Build history of the part. All positions in model axes, mm. A direction names the side the tool comes from. Give positions to 0.01 mm unless a question says otherwise; leave off trailing zeros. Write each loop counter-clockwise with the first axis right and the second up, starting at its lowest first coordinate (ties: lowest second). Pieces come first, ordered by that corner, then holes. Notation, with made-up numbers: (-36.75, 35) - (-27.75, 35) arc R22 ccw to (-27.75, 64) - close; hole circle Ø6 at (32, 54.5). An arc over 180 degrees is marked (long way). Use one line per item in the form item = value. Start each with the question number.
from build123d import *

# Parameters (mm, degrees)
BOSS_EXTRUDE1_DEPTH          = 18
F_4_0_4_DIAMETER_HOLE1_D     = 4
F_4_0_4_DIAMETER_HOLE1_DEPTH = 30
F_4_0_4_DIAMETER_HOLE1_TIP   = 1.201721238
F_4_0_4_DIAMETER_HOLE2_D     = 4
F_4_0_4_DIAMETER_HOLE2_DEPTH = 30
F_4_0_4_DIAMETER_HOLE2_TIP   = 1.201721238


with BuildPart() as part:
    # Sketch1 → Boss-Extrude1 (new body)
    with BuildSketch(Plane.XY):
        Polygon((30, 35), (60, 5), (60, -35), (-60, -35), (-60, 35), align=None)
    extrude(amount=BOSS_EXTRUDE1_DEPTH)

    # Ø4.0 (4) Diameter Hole1
    with Locations(Plane.ZY.offset(60)):
        with Locations((9, 16), (9, -16)):
            Hole(F_4_0_4_DIAMETER_HOLE1_D / 2, depth=F_4_0_4_DIAMETER_HOLE1_DEPTH)
            with Locations((0, 0, -(F_4_0_4_DIAMETER_HOLE1_DEPTH + F_4_0_4_DIAMETER_HOLE1_TIP / 2))):  # 118° drill point
                Cone(0, F_4_0_4_DIAMETER_HOLE1_D / 2, F_4_0_4_DIAMETER_HOLE1_TIP, mode=Mode.SUBTRACT)

    # Ø4.0 (4) Diameter Hole2
    with Locations(Plane(origin=(0, -35, 0), x_dir=(-1, 0, 0), z_dir=(0, -1, 0))):
        with Locations((-35, -9), (20, -9)):
            Hole(F_4_0_4_DIAMETER_HOLE2_D / 2, depth=F_4_0_4_DIAMETER_HOLE2_DEPTH)
            with Locations((0, 0, -(F_4_0_4_DIAMETER_HOLE2_DEPTH + F_4_0_4_DIAMETER_HOLE2_TIP / 2))):  # 118° drill point
                Cone(0, F_4_0_4_DIAMETER_HOLE2_D / 2, F_4_0_4_DIAMETER_HOLE2_TIP, mode=Mode.SUBTRACT)


solid = part.part
(1) Which spindle directions (+Z, -Z, +X, -X, +Y, -Y) get a long thin tool onto all of the face, cutting with end or side? Do faces 1 (the cylindrical face through (36.908, -19.79, 8.399)), 2 (the cylindrical face through (-45, -14, 9)), 3 (the flat face through (1, -35, 9)). Say none if no direction does.
(2) Pin check, flat tips, straight feed: pin 1 Ø6.5 at (y, z) = (16, 9) entering from -X; pin 2 Ø3 at (x, z) = (35, 9) entering from +Y; pin 3 Ø10 at (y, z) = (11.5, 6.5) entering from +X; pin 4 Ø6 at (y, z) = (25.5, 12.5) entering from +X. Stop position of each tip, or through.
(3) Two-plate mould, pull along Y, no slides. Class faces 4 (the cylindrical face through (-45, 18, 9)), 5 (the flat face through (60, -15, 9)), 6 (the conical face through (35.28, -4.01, 9.21)), 7 (the flat face through (-16, 35, 9)): +Y half, -Y half, draft (parallel to the pull), parting line (faces both ways), or undercut.
(4) Cut at B-B, the plane z = 4.5. Give the cut face in (x, y), then the cut area to 3 significant figures.
(5) Cut at A-A, the plane x = -40. Give the cut face in (y, z).
(6) Wall check: line 1 (Y direction, x = -45.75, z = 9); line 2 (X direction, y = -12.25, z = 9); line 3 (X direction, y = -15, z = 7.5). Give the ranges that are in metal, low to high. Write a range as from..to.
(7) Cut at D-D, the plane x = 51.5. Give the cut face in (y, z).
(8) Cut at C-C, the plane x = 39. Give the cut face in (y, z).
Solution:
q1.face_1 = -Y
q1.face_2 = -X
q1.face_3 = +Z, -Z, +X, -X, -Y
q2.pin_1 = -60
q2.pin_2 = 31.5
q2.pin_3 = 58.5
q2.pin_4 = 42.5
q3.face_4 = undercut
q3.face_5 = draft
q3.face_6 = -Y half
q3.face_7 = +Y half
q4.outline = (-60, -35) - (60, -35) - (60, 5) - (30, 35) - (-60, 35) - close
q4.area = 7,950 mm2
q5.outline = (-35, 0) - (35, 0) - (35, 18) - (-35, 18) - close; hole circle Ø4 at (-16, 9); hole circle Ø4 at (16, 9)
q6.line_1 = -35..-18, -14..14, 18..35
q6.line_2 = -60..-22, -18..33, 37..60
q6.line_3 = -29.88..-21.32, -18.68..33.68, 36.32..60
q7.outline = (-35, 0) - (13.5, 0) - (13.5, 18) - (-35, 18) - close
q8.outline = (-35, 0) - (26, 0) - (26, 18) - (-35, 18) - close
